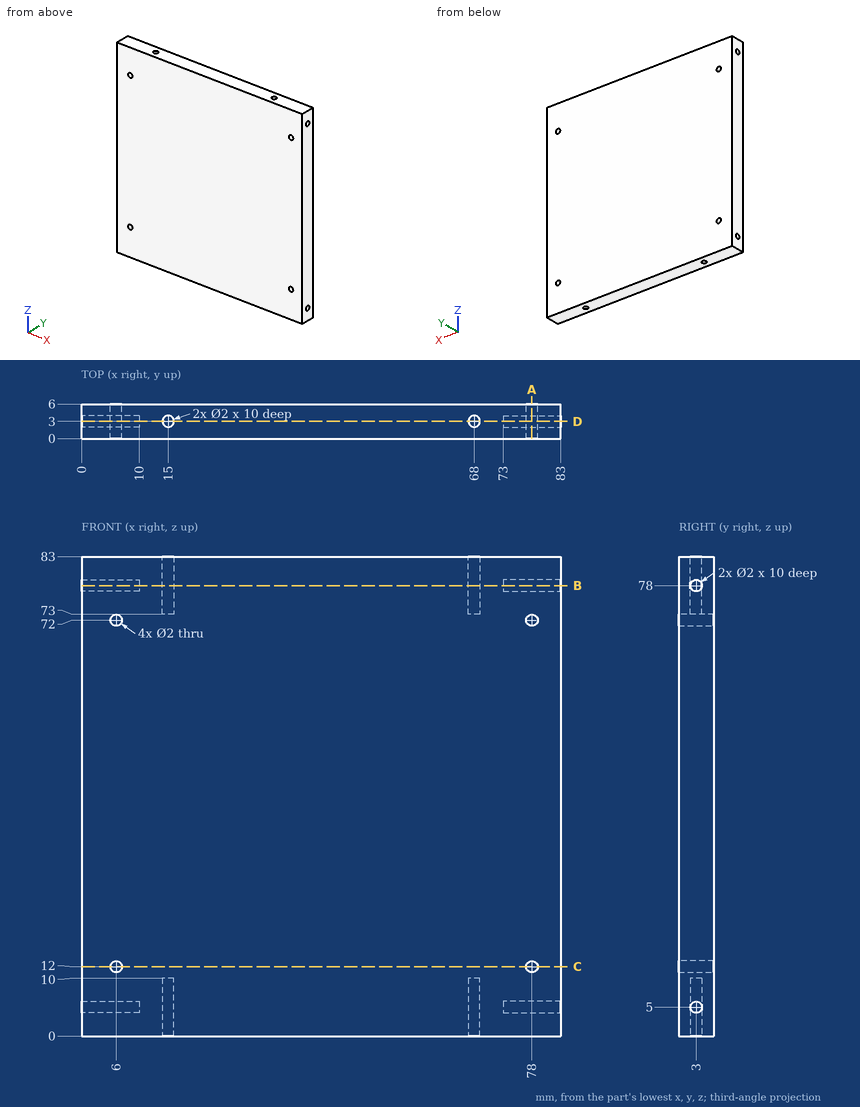
Answer from the drawing. Dimensions are ordinates in mm from the lowest x, y and z of the part. Give positions to 0.01 mm unless a question says otherwise; leave off trailing zeros. Write each loop counter-clockwise with the first axis right and the second up, starting at its lowest first coordinate (ties: lowest second). Pieces come first, ordered by that corner, then holes. Notation, with made-up numbers: (1, -15.75) -> (10, -15.75) arc R22 ccw to (10, 22.25) -> close; hole circle Ø1 at (30, 34.25). An arc over 180 degrees is marked (long way). Use a Markdown table: item, result.
(1) Section D-D, the plane y = 3 is taken. Give the number of separate pieces and of enclosed holes in the cut face, then the cut area to 3 significant figures.
Return value:
| item | result |
|---|---|
| separate pieces | 1 |
| enclosed holes | 4 |
| area | 6,720 mm2 |
(2) Find the intervals of material crossed by probe 1 along Z at (x, y) = (78, 3.2); probe 2 along X at (y, z) = (4.45, 72); probe 3 along Y at (x, z) = (15, 80), in increasing order. Write a range as from..to.
Return value:
| item | result |
|---|---|
| probe 1 | 0..4.02, 5.98..11, 13..71, 73..77.02, 78.98..83 |
| probe 2 | 0..5, 7..77, 79..83 |
| probe 3 | 0..2, 4..6 |
(3) Section C-C, the plane z = 12 is taken. Determine the outline of the cut face in (x, y), then the cut area to 3 significant figures.
Return value:
| item | result |
|---|---|
| outline | (0, 0) -> (5, 0) -> (5, 6) -> (0, 6) -> close; (7, 0) -> (77, 0) -> (77, 6) -> (7, 6) -> close; (79, 0) -> (83, 0) -> (83, 6) -> (79, 6) -> close |
| area | 474 mm2 |
(4) Section B-B, the plane z = 78 is taken. Determine the outline of the cut face in (x, y), then the cut area to 3 significant figures.
Return value:
| item | result |
|---|---|
| outline | (0, 0) -> (83, 0) -> (83, 2) -> (73, 2) -> (73, 4) -> (83, 4) -> (83, 6) -> (0, 6) -> (0, 4) -> (10, 4) -> (10, 2) -> (0, 2) -> close; hole circle Ø2 at (15, 3); hole circle Ø2 at (68, 3) |
| area | 452 mm2 |
(5) Section A-A, the plane x = 78 is taken. Determine the outline of the cut face in (y, z), then the cut area to 3 significant figures.
Return value:
| item | result |
|---|---|
| outline | (0, 0) -> (6, 0) -> (6, 11) -> (0, 11) -> close; (0, 13) -> (6, 13) -> (6, 71) -> (0, 71) -> close; (0, 73) -> (6, 73) -> (6, 83) -> (0, 83) -> close; hole circle Ø2 at (3, 5); hole circle Ø2 at (3, 78) |
| area | 468 mm2 |
(6) Flat-ended cylindrical pins translate along their axes: P1, Ø0.6, axis at x = 15, y = 3, coming from the +Z side; P2, Ø1.6, axis at x = 15, y = 3, coming from the -Z side; P3, Ø1.6, axis at y = 3, z = 78, coming from the +X side. Find the tip coordinate at first contact, or state that the pin passes through.
Return value:
| item | result |
|---|---|
| P1 | z = 73 |
| P2 | z = 10 |
| P3 | x = 73 |
